Input: part model. Units: mm. Frame: model coordinates. Round coordinates to 2 decimals unless told otherwise and drop trailing zeros. Order: outer loops, then holes, each group sorted by start corner. A loop starts at its lowest first (then second) coordinate and runs counter-clockwise, first axis right, second up. Notation, with made-up numbers: (27, 77) -> (31, 77) arc R23 cw to (31, 96) -> close; hole circle Ø5 at (-1.5, -18.5). An arc over 180 degrees is marked (long way). Use a Markdown table: item, result.
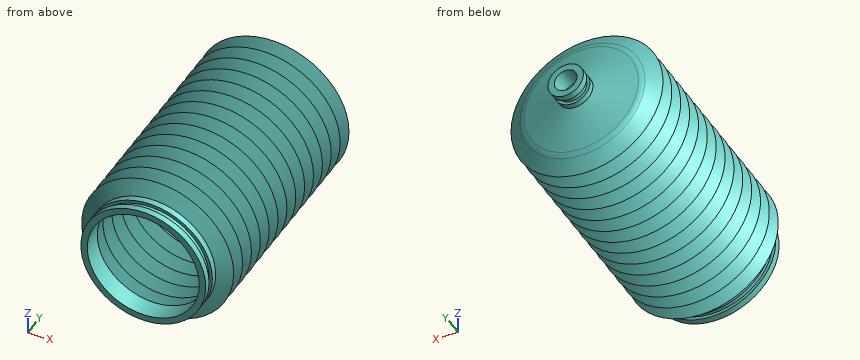
Autodesk Inventor part; units mm, degrees
ref_plane "YZ Plane" through (0, 0, 0) normal (1, 0, 0) x (0, 1, 0)
ref_plane "XZ Plane" through (0, 0, 0) normal (0, 1, 0) x (-1, 0, 0)
ref_plane "XY Plane" through (0, 0, 0) normal (0, 0, 1) x (1, 0, 0)
sketch "Sketch2" plane through (0, 0, 0) normal (0, 0, 1) x (1, 0, 0)
  line L0 (37, 65.25) -> (-37, 65.25)
  line L1 (-9, 234.5) -> (9, 234.5)
  point P0 (0, 0)
  dimension "d47" = 169.25
sketch "Sketch1" plane through (0, 0, 0) normal (0, 0, 1) x (1, 0, 0)
  line L0 (-36.7449, 53.25) -> (37.2551, 53.25)
  line L1 (35, 65.25) -> (35, 53.25)
  line L2 (7.056, 234.5) -> (7.056, 222.5)
  line L3 (7.056, 234.5) -> (7.056, 222.5)
  line L4 (7.056, 234.5) -> (11.056, 234.5)
  line L5 (35, 53.25) -> (39, 53.25)
  line L6 (39, 53.25) -> (39, 57.25)
  line L7 (39, 57.25) -> (37, 57.25)
  line L8 (37, 57.25) -> (37, 61.25)
  line L9 (37, 61.25) -> (39, 61.25)
  line L10 (39, 61.25) -> (39, 65.25)
  line L11 (39, 65.25) -> (37, 65.25) construction
  line L12 (11.056, 234.5) -> (11.056, 230.5)
  line L13 (11.056, 230.5) -> (9.056, 230.5)
  line L14 (9.056, 230.5) -> (9.056, 226.5)
  line L15 (9.056, 226.5) -> (11.056, 226.5)
  line L16 (11.056, 226.5) -> (11.056, 223.0191)
  line L17 (39, 65.25) -> (47.4666, 70.5714)
  line L18 (37, 65.25) -> (45.4666, 70.5714)
  line L19 (37, 65.25) -> (37, 83.6946) construction
  line L20 (45.4666, 70.5714) -> (37, 70.5714) construction
  line L21 (45.4666, 70.5714) -> (37, 75.8928)
  line L22 (47.4666, 70.5714) -> (39, 75.8928)
  line L23 (37, 75.8928) -> (46.5513, 75.8928) construction
  line L24 (45.4666, 81.2141) -> (37, 86.5355)
  line L25 (47.4666, 81.2141) -> (39, 86.5355)
  line L26 (39, 75.8928) -> (47.4666, 81.2141)
  line L27 (37, 75.8928) -> (45.4666, 81.2141)
  line L28 (45.4666, 91.8569) -> (37, 97.1783)
  line L29 (47.4666, 91.8569) -> (39, 97.1783)
  line L30 (39, 86.5355) -> (47.4666, 91.8569)
  line L31 (37, 86.5355) -> (45.4666, 91.8569)
  line L32 (45.4666, 102.4996) -> (37, 107.821)
  line L33 (47.4666, 102.4996) -> (39, 107.821)
  line L34 (39, 97.1783) -> (47.4666, 102.4996)
  line L35 (37, 97.1783) -> (45.4666, 102.4996)
  line L36 (45.4666, 113.1424) -> (37, 118.4638)
  line L37 (47.4666, 113.1424) -> (39, 118.4638)
  line L38 (39, 107.821) -> (47.4666, 113.1424)
  line L39 (37, 107.821) -> (45.4666, 113.1424)
  line L40 (45.4666, 123.7851) -> (37, 129.1065)
  line L41 (47.4666, 123.7851) -> (39, 129.1065)
  line L42 (39, 118.4638) -> (47.4666, 123.7851)
  line L43 (37, 118.4638) -> (45.4666, 123.7851)
  line L44 (45.4666, 134.4279) -> (37, 139.7493)
  line L45 (47.4666, 134.4279) -> (39, 139.7493)
  line L46 (39, 129.1065) -> (47.4666, 134.4279)
  line L47 (37, 129.1065) -> (45.4666, 134.4279)
  line L48 (45.4666, 145.0706) -> (37, 150.392)
  line L49 (47.4666, 145.0706) -> (39, 150.392)
  line L50 (39, 139.7493) -> (47.4666, 145.0706)
  line L51 (37, 139.7493) -> (45.4666, 145.0706)
  line L52 (45.4666, 155.7134) -> (37, 161.0348)
  line L53 (47.4666, 155.7134) -> (39, 161.0348)
  line L54 (39, 150.392) -> (47.4666, 155.7134)
  line L55 (37, 150.392) -> (45.4666, 155.7134)
  line L56 (45.4666, 166.3561) -> (37, 171.6775)
  line L57 (47.4666, 166.3561) -> (39, 171.6775)
  line L58 (39, 161.0348) -> (47.4666, 166.3561)
  line L59 (37, 161.0348) -> (45.4666, 166.3561)
  line L60 (45.4666, 176.9989) -> (37, 182.3203)
  line L61 (47.4666, 176.9989) -> (39, 182.3203)
  line L62 (39, 171.6775) -> (47.4666, 176.9989)
  line L63 (37, 171.6775) -> (45.4666, 176.9989)
  line L64 (45.4666, 187.6417) -> (37, 192.963)
  line L65 (47.4666, 187.6417) -> (39, 192.963)
  line L66 (39, 182.3203) -> (47.4666, 187.6417)
  line L67 (37, 182.3203) -> (45.4666, 187.6417)
  line L68 (0, -37.6229) -> (0, 264.2373)
  line L69 (9.056, 222.5) -> (7.056, 222.5)
  line L70 (37, 65.25) -> (35, 65.25)
  line L71 (0, 208431.7305) -> (0, -209414.2305)
  line L72 (37, 65.25) -> (-37, 65.25)
  line L73 (37, 65.25) -> (-37, 65.25) construction
  line L74 (37, 65.25) -> (35, 65.25)
  line L75 (7.056, 222.5) -> (9.056, 222.5)
  line L76 (11.056, 223.0191) -> (7.056, 224.2003)
  line L77 (45.4666, 198.2844) -> (37, 203.6058)
  line L78 (47.4666, 198.2844) -> (39, 203.6058)
  line L79 (39, 192.963) -> (47.4666, 198.2844)
  line L80 (37, 192.963) -> (45.4666, 198.2844)
  line L81 (45.4666, 208.9272) -> (37, 214.2485)
  line L82 (47.4666, 208.9272) -> (39, 214.2485)
  line L83 (39, 203.6058) -> (47.4666, 208.9272)
  line L84 (37, 203.6058) -> (45.4666, 208.9272)
  line L85 (9.056, 222.5) -> (37, 214.2485)
  line L86 (7.056, 224.2003) -> (35.6774, 215.7488)
  arc A0 (39, 214.2485) -> (35.6774, 215.7488) centre (31.8976, 202.9482) ccw
  point P0 (0, 0)
  point P1 (39, 75.8928)
  point P2 (39, 86.5355)
  point P3 (39, 97.1783)
  point P4 (39, 107.821)
  point P5 (39, 118.4638)
  point P6 (39, 129.1065)
  point P7 (39, 139.7493)
  point P8 (39, 150.392)
  point P9 (39, 161.0348)
  point P10 (39, 171.6775)
  point P11 (39, 182.3203)
  point P12 (7, 203.6144)
  point P13 (39, 192.963)
  point P14 (9, 223.6095)
  point P15 (9, 222.5)
  point P16 (11.056, 223.0191)
  dimension "d0" = 4
  dimension "d1" = 12
  dimension "d2" = 4
  dimension "d3" = 2
  dimension "d4" = 2
  dimension "d5" = 4
  dimension "d7" = 2
  dimension "d8" = 2
  dimension "d12" = 122.15
  dimension "d13" = 1.0643
  dimension "d17" = 10
  dimension "d18" = 10.6427
  dimension "d28" = 10.6427
  dimension "d34" = 12
  dimension "d37" = 7.056
  dimension "d39" = 169.25
  dimension "d46" = 2
  dimension "d48" = 1.0643
  dimension "d49" = 4
revolve "Revolution1" add sketch "Sketch1" angle 360 about axis through (0, -37.6229, 0) along (0, 1, 0) contours L1 L70 L18 L21 L27 L24 L31 L28 L35 L32 L39 L36 L43 L40 L47 L44 L51 L48 L55 L52 L59 L56 L63 L60 L67 L64 L80 L77 L84 L81 L85 L69 L2 L76 L86 A0 L82 L83 L78 L79 L65 L66 L61 L62 L57 L58 L53 L54 L49 L50 L45 L46 L41 L42 L37 L38 L33 L34 L29 L30 L25 L26 L22 L17 L10 L9 L8 L7 L6 L5 L0 | L2 L4 L12 L13 L14 L15 L16 L76
equation "\"d0\" = 0.333333 * d1"
equation "\"d2\" = d0"
equation "\"d5\" = d0"
equation "\"d37\" = RevolveDIA"
equation "\"d10\" = d9"
properties part number "MCEN4000:T7" material "RUBBER, SILICONE"
1) Ray query, probe 1 along X at (y, z) = (60.75, 0); probe 2 along X at (y, z) = (56, 0); probe 3 along Z at (x, y) = (0, 231). Return the intervals inside material, ascending.
Answer key:
| item | result |
|---|---|
| probe 1 | x = -37 to -35, 35 to 37 |
| probe 2 | x = -39 to -35, 35 to 39 |
| probe 3 | z = -11.06 to -7.06, 7.06 to 11.06 |
2) Cut plane A-A on y = 185.5. Return loops of the section in (x, z), and give its area (3 significant figures).
Answer key:
| item | result |
|---|---|
| outline | circle Ø88.12 at (0, 0); hole circle Ø84.12 at (0, 0) |
| area | 541 mm^2 |
3) Contact query for flat-ended pins moving along their axis: P1, Ø6.5, axis at x = 5, z = -2, coming from the -Y side; P2, Ø1.5, axis at x = 24, z = 33, coming from the -Y side; P3, Ø3, axis at y = 77, z = -11, coming from the +X side. Output: stop coordinate, or through.
Answer key:
| item | result |
|---|---|
| P1 | stops at y = 222.5 |
| P2 | stops at y = 65.91 |
| P3 | stops at x = 41.75 |
